```python
from build123d import *

# Parameters (mm, degrees)
BOSS_EXTRUDE1_DEPTH = 1.6
SKETCH2_R           = 1
CUT_EXTRUDE1_DEPTH  = 60.868490043
FILLET1_R           = 0.5
CUT_EXTRUDE3_DEPTH  = 0.8
FILLET2_R           = 0.4


with BuildPart() as part:
    # Sketch1 → Boss-Extrude1 (new body)
    with BuildSketch(Plane.XY):
        with BuildLine():
            Line((3.78, 5.348981211), (3.78, 25.241675085))
            Line((3.78, 25.241675085), (0, 28.81))
            Line((0, 28.81), (1.140731522, 48.297942259))
            ThreePointArc((1.140731522, 48.297942259), (2.179202609, 54.012368785), (4.56, 59.31))
            Line((4.56, 59.31), (4.56, 37.74))
            Line((4.56, 37.74), (5.78, 36.52))
            Line((5.78, 36.52), (5.78, 12.266686594))
            ThreePointArc((5.78, 12.266686594), (6.339471549, 6.033709777), (8, 0))
            ThreePointArc((8, 0), (4.962014359, 1.942369992), (3.78, 5.348981211))
        make_face()
    extrude(amount=BOSS_EXTRUDE1_DEPTH)

    # Sketch2 → Cut-Extrude1 (cut, through all)
    with BuildSketch(Plane.XY.offset(1.6)):
        with Locations((3.5, 31.95)):
            Circle(SKETCH2_R)
    extrude(amount=-CUT_EXTRUDE1_DEPTH, mode=Mode.SUBTRACT)

    # Fillet1
    fillet1_edges = [part.edges().sort_by_distance(p)[0] for p in [
        (3.78, 25.241675085, 0.8),
        (0, 28.81, 0.8),
        (4.56, 37.74, 0.8),
        (5.78, 36.52, 0.8),
        (8, 0, 0.8),
    ]]
    fillet(fillet1_edges, radius=FILLET1_R)

    # Sketch8 → Cut-Extrude3 (cut)
    with BuildSketch(Plane(origin=(0, 0, 0), x_dir=(-1, 0, 0), z_dir=(0, 0, -1))):
        Polygon((-2.943771792, 26.031075601), (11.550433579, 26.031075601), (11.550433579, 65.314635105), (-14.375020628, 65.314635105), (-14.375020628, 34.529960463), align=None)
    extrude(amount=-CUT_EXTRUDE3_DEPTH, mode=Mode.SUBTRACT)

    # Fillet2
    fillet2_edges = [part.edges().sort_by_distance(p)[0] for p in [
        (4.361885896, 27.085412591, 0.8),
        (4.361885896, 27.085412591, 0),
    ]]
    fillet(fillet2_edges, radius=FILLET2_R - 0.0001)  # a hair under: the kernel refuses the full size


solid = part.part
```
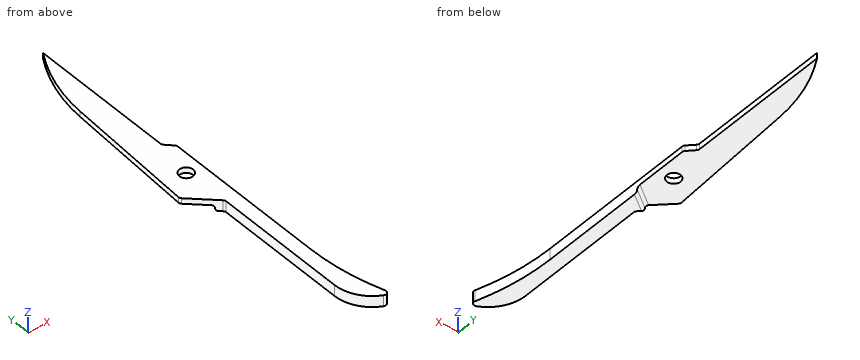
Model file for the job. Use its own axes, mm. Coordinates: 2 decimals unless noted, no trailing zeros. Write each loop counter-clockwise with the first axis right and the second up, starting at its lowest first coordinate (ties: lowest second). Pieces come first, ordered by that corner, then holes. Notation, with made-up numbers: (82.25, 31.5) - (98.25, 31.5) arc R17 cw to (98.25, 63.5) - close; hole circle Ø3 at (34, -12.75). An arc over 180 degrees is marked (long way). Use a Markdown table: item, result. Add a question column.
Item 1: Drop flat-ended pins along their axis: pin 1 (0.8 mm diameter, centred on y = 14.5, z = 0.5, fed in from -X); pin 2 (4.5 mm diameter, centred on x = 2.5, y = 37, fed in from -Z); pin 3 (0.8 mm diameter, centred on y = 20.5, z = 1, fed in from +X). Give the stop position or say it passes through.
Item 2: Drill centre lines: line 1 along Z through (x, y) = (2.25, 37.5); line 2 along Y through (x, z) = (3.5, 1.4); line 3 along X through (y, z) = (29, 1.1). Where is each one in solid material? Low to high.
Item 3: Band-saw the part on A-A, the plane y = 31.95. Write the cut outline in (x, z).
Item 4: Band-saw the part on B-B, the plane y = 13. Write the cut outline in (x, z), and give its area (3 significant figures).
Item 5: Band-saw the part on C-C, the plane x = 1.75. Write the cut outline in (y, z).
A:
| question | item | result |
|---|---|---|
| 1 | pin 1 | stops at x = 3.78 |
| 1 | pin 2 | stops at z = 0.8 |
| 1 | pin 3 | stops at x = 5.78 |
| 2 | line 1 | z = 0.8 to 1.6 |
| 2 | line 2 | y = 25.51 to 30.95, 32.95 to 57.36 |
| 2 | line 3 | x = 0.01 to 5.78 |
| 3 | outline | (0.18, 0.8) - (2.5, 0.8) - (2.5, 1.6) - (0.18, 1.6) - close; (4.5, 0.8) - (5.78, 0.8) - (5.78, 1.6) - (4.5, 1.6) - close |
| 4 | outline | (3.78, 0) - (5.78, 0) - (5.78, 1.6) - (3.78, 1.6) - close |
| 4 | area | 3.20 mm² |
| 5 | outline | (27.16, 0.8) - (52.44, 0.8) - (52.44, 1.6) - (27.16, 1.6) - close |
